For this review, take the finished solid that the model builds, in its own axes (mm). Face numbers are marked on the shaded views. Round coordinates to 2 decimals unless told otherwise and drop trailing zeros. Order: outer loops, then holes, each group sorted by start corner. A loop starts at its lowest first (then second) coordinate and runs counter-clockwise, first axis right, second up. Notation, with made-up numbers: (40, 57) - (49, 57) arc R23 cw to (49, 91) - close; hole circle Ø2 at (13.25, 86). An arc over 180 degrees is marked (long way). One line per question, with ' | ' between items.
```python
from build123d import *

# Parameters (mm, degrees)
SKETCH1_R              = 3.175
BOSS_EXTRUDE1_DEPTH    = 6.35
F_10_32_TAPPED_HOLE1_D = 4.0386


with BuildPart() as part:
    # Sketch1 → Boss-Extrude1 (new body)
    with BuildSketch(Plane(origin=(0, 0, 0), x_dir=(1, 0, 0), z_dir=(0, 1, 0))):
        with BuildLine():
            Line((6.35, 24), (6.35, 0))
            ThreePointArc((6.35, 0), (0, -6.35), (-6.35, 0))
            Line((-6.35, 0), (-6.35, 24))
            ThreePointArc((-6.35, 24), (0, 30.35), (6.35, 24))
        make_face()
        Circle(SKETCH1_R, mode=Mode.SUBTRACT)
    extrude(amount=BOSS_EXTRUDE1_DEPTH)

    # #10-32 Tapped Hole1 (through all)
    with Locations(Plane(origin=(0, 6.35, 0), x_dir=(1, 0, 0), z_dir=(0, 1, 0))):
        with Locations((0, 24)):
            Hole(F_10_32_TAPPED_HOLE1_D / 2)


solid = part.part
```
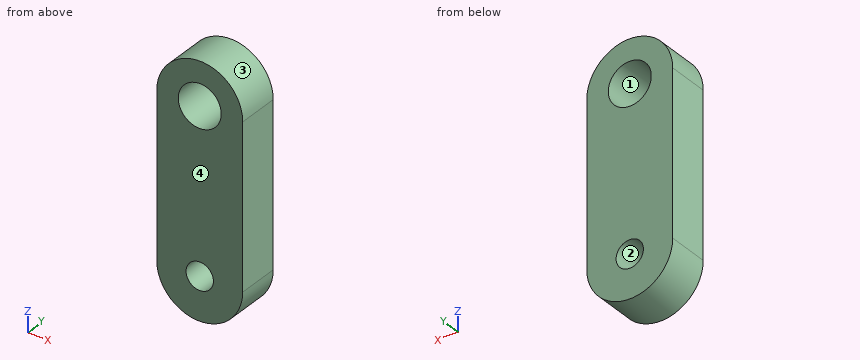
(1) For probe 1 along Z at (x, y) = (0, 4.5) (3 decimals); probe 2 along X at (y, z) = (1.75, -24); probe 3 along Z at (x, y) = (-0.5, 2.75), list the stretches that pass through material, from the lowest coordinate up. Write a range as [from, to].
Output values:
probe 1: [-30.35, -26.019], [-21.981, -3.175], [3.175, 6.35] | probe 2: [-6.35, -2.02], [2.02, 6.35] | probe 3: [-30.33, -25.96], [-22.04, -3.14], [3.14, 6.33]
(2) We need section B-B on y = 0.5. State the section outline as (x, z) points (3 decimals).
Output values:
outline: (-6.35, -24) arc R6.35 ccw to (6.35, -24) - (6.35, 0) arc R6.35 ccw to (-6.35, 0) - close; hole circle Ø6.35 at (0, 0); hole circle Ø4.039 at (0, -24)
(3) We need section D-D on x = 2.75. State the section outline as (y, z) points.
Output values:
outline: (0, -29.72) - (6.35, -29.72) - (6.35, -1.59) - (0, -1.59) - close; (0, 1.59) - (6.35, 1.59) - (6.35, 5.72) - (0, 5.72) - close
(4) Insertion check: pin 1 (3 mm diameter, centred on x = -3.5, y = 4.5, fed in from -Z); pin 2 (2 mm diameter, centred on x = 3.5, y = 1.5, fed in from -Z). Each pin has a flat end and moves straight along its axis. Give the tip position at first contact, or say it passes through.
Output values:
pin 1: z = -30.03 | pin 2: z = -29.84
(5) Mouldability with a two-part tool opening along Z and no side actions: class the marked faces 1, 2, 3 and 4 as released by +Z, released by -Z, zero draft, split by the parting line, or undercut.
Output values:
face 1: undercut | face 2: undercut | face 3: released by +Z | face 4: zero draft
(6) We need section C-C on z = -23. State the section outline as (x, y) points.
Output values:
outline: (-6.35, 0) - (-1.75, 0) - (-1.75, 6.35) - (-6.35, 6.35) - close; (1.75, 0) - (6.35, 0) - (6.35, 6.35) - (1.75, 6.35) - close
(7) We need section A-A on x = 0. State the section outline as (y, z) points (3 decimals).
Output values:
outline: (0, -30.35) - (6.35, -30.35) - (6.35, -26.019) - (0, -26.019) - close; (0, -21.981) - (6.35, -21.981) - (6.35, -3.175) - (0, -3.175) - close; (0, 3.175) - (6.35, 3.175) - (6.35, 6.35) - (0, 6.35) - close
